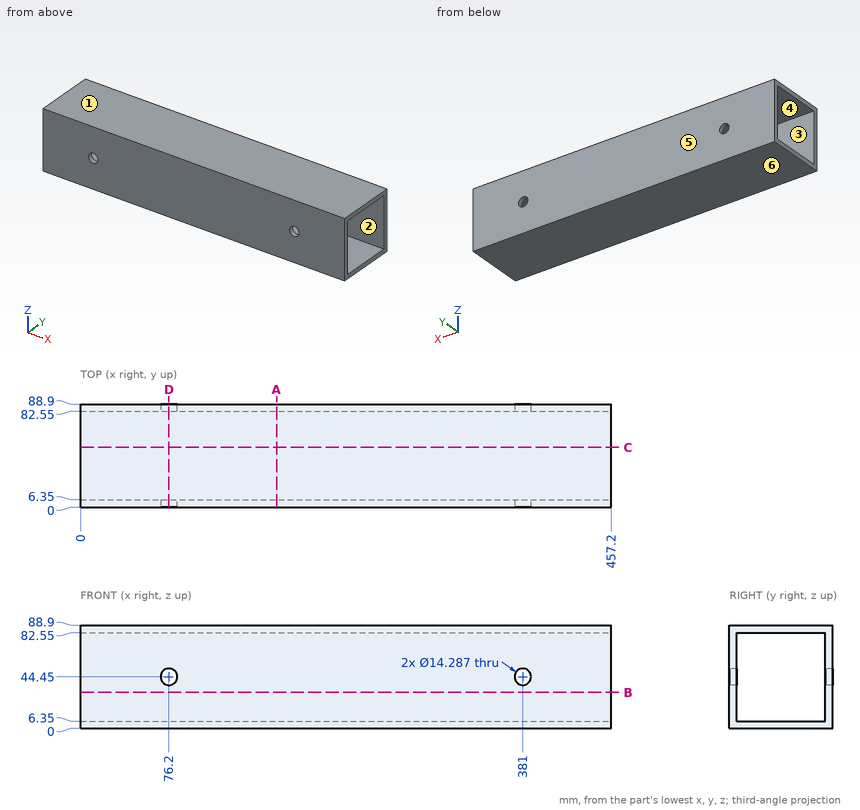
For this review, use the dimensioned drawing (mm, ordinates from the lowest corner) and the shaded views. A direction names the side the tool comes from. Coordinates: 2 decimals unless noted, no trailing zeros. Order: outer loops, then holes, each group sorted by start corner. A loop starts at its lowest first (then second) coordinate and runs counter-clockwise, first axis right, second up. Notation, with made-up numbers: M 84.5,74.5 L 136.5,74.5 A10 ccw 136.5,88.5 Z; hole C 36.5,-24 d2. An arc over 180 degrees is marked long. Answer as a JSON object with one key per item and string values. Group by question number.
1) Tool access review of the marked faces 1 and 2: name each direction out of +Z, -Z, +X, -X, +Y, -Y from which nothing blocks a thin tool from reaching the whole face with its end or side.
2) Wall thickness on L1, parallel to Y at x = 26.5, z = 73; L2, parallel to Z at x = 76.2, y = 4.5: over which ranges is each line inside the solid? List them lowest first.
3) For pin 1 (16.5 mm diameter, centred on x = 381, z = 44.45, fed in from -Y); pin 2 (8.5 mm diameter, centred on x = 76.2, z = 44.45, fed in from -Y), all flat-tipped, find the tip position at first contact; note any pin that passes through.
4) Add section B-B, the plane z = 31. Write out the cut boundary in (x, y).
5) Mouldability with a two-part tool opening along Z and no side actions: class the marked faces 3, 4, 5 and 6 as pulls with the +Z half, pulls with the -Z half, needs draft (parallel to the pull), parting line crosses it, or undercut.
6) Add section A-A, the plane x = 169. Write out the cut boundary in (y, z).
7) Add section D-D, the plane x = 76.2. Write out the cut boundary in (y, z).
Computed values:
{
 "1": {"face 1": "+Z, +X, -X, +Y, -Y", "face 2": "+X, -X"},
 "2": {"L1": "y = 0 to 6.35, 82.55 to 88.9", "L2": "z = 0 to 37.31, 51.59 to 88.9"},
 "3": {"pin 1": "stops at y = 0", "pin 2": "passes through"},
 "4": {"outline": "M 0,0 L 457.2,0 L 457.2,6.35 L 0,6.35 Z; M 0,82.55 L 457.2,82.55 L 457.2,88.9 L 0,88.9 Z"},
 "5": {"face 3": "undercut", "face 4": "undercut", "face 5": "needs draft", "face 6": "pulls with the -Z half"},
 "6": {"outline": "M 0,0 L 88.9,0 L 88.9,88.9 L 0,88.9 Z; hole M 6.35,6.35 L 82.55,6.35 L 82.55,82.55 L 6.35,82.55 Z"},
 "7": {"outline": "M 0,0 L 88.9,0 L 88.9,37.31 L 82.55,37.31 L 82.55,6.35 L 6.35,6.35 L 6.35,37.31 L 0,37.31 Z; M 0,51.59 L 6.35,51.59 L 6.35,82.55 L 82.55,82.55 L 82.55,51.59 L 88.9,51.59 L 88.9,88.9 L 0,88.9 Z"}
}
